```python
from build123d import *

# Parameters (mm, degrees)
F0_W     = 109.595508
F0_H     = 83.483816
F1_DEPTH = 25.4
F2_R     = 20.651308
F3_DEPTH = 25.4
F5_DEPTH = 25.4


with BuildPart() as f1:
    # F0 (on Front) → F1 (new body)
    with BuildSketch(Plane.XZ):
        Rectangle(F0_W, F0_H)
    extrude(amount=F1_DEPTH)

    # F2 (on face) → F3 (join)
    with BuildSketch(Plane.XZ.offset(25.4)):
        Circle(F2_R)
    extrude(amount=F3_DEPTH)

    # F4 (on Right) → F5 (cut, symmetric)
    with BuildSketch(Plane.YZ):
        Polygon((-65.909445, 37.025604), (-65.909445, -38.188711), (-35.280939, 37.025604), align=None)
    extrude(amount=F5_DEPTH, both=True, mode=Mode.SUBTRACT)


solid = f1.part
```
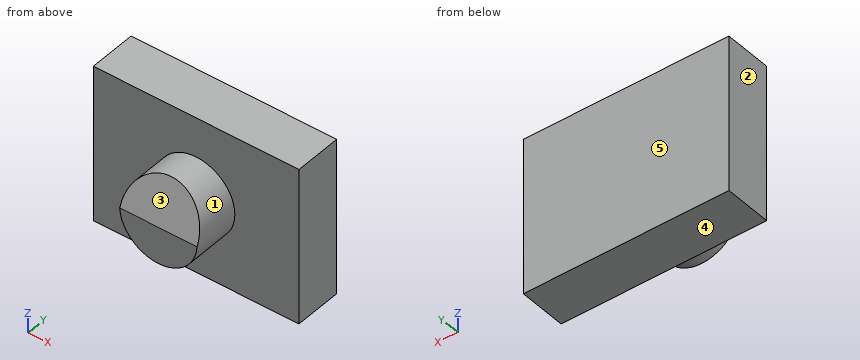
Design review of the part built by this model. Coordinates are the model's own, in mm. Face numbers are marked on the shaded views. A direction names the side the tool comes from. Give positions to 0.01 mm unless a question says otherwise; leave off trailing zeros. Order: outer loops, then holes, each group sorted by start corner. A loop starts at its lowest first (then second) coordinate and runs counter-clockwise, first axis right, second up. Notation, with made-up numbers: (71.5, -24) - (85.5, -24) arc R22 cw to (85.5, 2) - close; hole circle Ø6 at (84.5, 86.5). An arc over 180 degrees is marked (long way). Use a Markdown table: item, result. Add a question column.
(1) Machinability: for the marked faces 1 and 2, which of the approach directions +Z, -Z, +X, -X, +Y, -Y give a long, thin tool a straight path to every point of the face, cutting with its end or side? Answer none if there is none.
(2) Add section C-C on y = -34. Give the boundary of the cut face in (x, z), then the cut area to 3 significant figures.
(3) Add section A-A on x = 0. Give the boundary of the cut face in (y, z).
(4) Mouldability with a two-part tool opening along Y and no side actions: class the marked faces 3, 4 and 5 as +Y half, -Y half, draft (parallel to the pull), parting line (faces both ways), or undercut.
(5) Clearance check with flat-ended pins moving along their axes: P1, Ø1, axis at x = 23.5, z = -0.5, coming from the -Y side; P2, Ø3, axis at x = -7, y = -43, coming from the +Z side. State where each tip first meets the part, or that it passes through.
(6) Add section B-B on z = 14. Give the boundary of the cut face in (x, y), then the cut area to 3 significant figures.
(7) Add section D-D on x = 30.5. Give the boundary of the cut face in (y, z).
(8) Wall thickness on probe 1 along Y at (x, z) = (-36, 33); probe 2 along Z at (x, y) = (1, -30); probe 3 along X at (y, z) = (-37, -9): over which ranges is each line inside the solid? List them lowest first. Write a range as [from, to].
Report:
| question | item | result |
|---|---|---|
| 1 | face 1 | -Y |
| 1 | face 2 | +Z, -Z, -X, +Y, -Y |
| 2 | outline | circle Ø41.3 at (0, 0) |
| 2 | area | 1,340 mm² |
| 3 | outline | (-50.8, -20.65) - (-25.4, -20.65) - (-25.4, -41.74) - (0, -41.74) - (0, 41.74) - (-25.4, 41.74) - (-25.4, 20.65) - (-41.95, 20.65) - (-50.8, -1.08) - close |
| 4 | face 3 | -Y half |
| 4 | face 4 | draft |
| 4 | face 5 | +Y half |
| 5 | P1 | stops at y = -25.4 |
| 5 | P2 | stops at z = 19.85 |
| 6 | outline | (-54.8, -25.4) - (-15.18, -25.4) - (-15.18, -44.66) - (15.18, -44.66) - (15.18, -25.4) - (54.8, -25.4) - (54.8, 0) - (-54.8, 0) - close |
| 6 | area | 3,370 mm² |
| 7 | outline | (-25.4, -41.74) - (0, -41.74) - (0, 41.74) - (-25.4, 41.74) - close |
| 8 | probe 1 | y = [-25.4, 0] |
| 8 | probe 2 | z = [-20.63, 20.63] |
| 8 | probe 3 | x = [-18.59, 18.59] |
